Autodesk Inventor part; units mm, degrees
ref_plane "YZ Plane" through (0, 0, 0) normal (1, 0, 0) x (0, 1, 0)
ref_plane "XZ Plane" through (0, 0, 0) normal (0, 1, 0) x (-1, 0, 0)
ref_plane "XY Plane" through (0, 0, 0) normal (0, 0, 1) x (1, 0, 0)
sketch "Skizze1" plane through (0, 0, 0) normal (0, 0, 1) x (1, 0, 0)
  line L0 (0, 0) -> (0, 5.7)
  line L1 (0, 5.7) -> (-2.3, 5.7)
  line L2 (-2.3, 5.7) -> (-2.3, 1.71)
  line L3 (-2.3, 1.71) -> (-1.75, 1.71)
  line L4 (-1.75, 1.71) -> (-1.75, 0.855)
  line L5 (-1.75, 0.855) -> (-1.95, 0.855)
  line L6 (-1.95, 0.855) -> (-1.95, 0)
  line L7 (-1.95, 0) -> (0, 0)
  dimension "d0" = 4.6
  dimension "d1" = 5.7
  dimension "d2" = 3.9
  dimension "d3" = 0.2
  dimension "d4" = 3.99
revolve "Umdrehung1" add sketch "Skizze1" angle 360 about axis through (0, 0, 0) along (0, 1, 0)
sketch "Skizze2" plane through (0, 5.7, 0) normal (0, 1, 0) x (1, 0, 0)
  circle A0 centre (0, 0) radius 2.3
hole "Bohrung1" at (0, 5.7, 0) direction (0, -1, 0) diameter 2.459 end through all
chamfer "Fase1" distance 0.3 angle 45 4 edges at (0, 5.7, -1.2295) (1.95, 0, 0) (0, 0, -1.2295) (2.3, 5.7, 0)
equation "\"d4\" = 0.7 * d1"
properties part number "RX-M3x5,7" material "Messing, weicher Gelbton"
Work out the finished part from the listing and answer in its coordinate system (mm). A direction names the side the tool comes from. Round coordinates to 2 decimals unless told otherwise and drop trailing zeros. Write each loop counter-clockwise with the first axis right and the second up, starting at its lowest first coordinate (ties: lowest second). Pieces come first, ordered by that corner, then holes.
1) The mould has two halves that part along Z. Classify faces 3 (the flat face through (0, 1.71, 2)), 4 (the cylindrical face through (0.748, 2.814, -0.976)), 5 (the cylindrical face through (-1.617, 1.277, 0.67)): pulls with the +Z half, pulls with the -Z half, needs draft (parallel to the pull), parting line crosses it, or undercut.
2) A cutting plane is placed at D-D (y = 4.2). Give the vertices of the cut face in (x, z), plus the area to 3 significant figures.
3) A tool of negligible diameter and unlimited length cuts with its end or side. For faces 1 (the cylindrical face through (1.825, 3.529, 1.4)), 2 (the cylindrical face through (1.437, 0.574, -1.318)), from which of +Z, -Z, +X, -X, +Y, -Y can it reach the whole face along a straight path? Write none if from no direction.
4) Straight lines are drawn through the part: line 1 (Z direction, x = 0, y = 4.2); line 2 (Z direction, x = -0.55, y = 3.8); line 3 (X direction, y = 3.5, z = 0.5) (3 decimals). For each, find the intervals that lie inside material, in ascending order.
5) Given pin 1 Ø2 at (x, z) = (0, -0.5) entering from +Y, flat-ended and moving along its own axis, determine where the tip first touches the part or whether it passes through.
6) A cutting plane is placed at C-C (y = 0.4). Give the vertices of the cut face in (x, z).
Completed:
1. face 3: needs draft
1. face 4: undercut
1. face 5: parting line crosses it
2. outline: circle Ø4.6 at (0, 0); hole circle Ø2.46 at (0, 0)
2. area: 11.9 mm2
3. face 1: +Y, -Y
3. face 2: -Y
4. line 1: z = -2.3 to -1.23, 1.23 to 2.3
4. line 2: z = -2.23 to -1.1, 1.1 to 2.23
4. line 3: x = -2.245 to -1.123, 1.123 to 2.245
5. pin 1: stops at y = 5.67
6. outline: circle Ø3.9 at (0, 0); hole circle Ø2.46 at (0, 0)
